Build history of the part. All positions in model axes, mm. A direction names the side the tool comes from. Coordinates: 2 decimals unless noted, no trailing zeros. Order: outer loops, then holes, each group sorted by start corner. A loop starts at its lowest first (then second) coordinate and runs counter-clockwise, first axis right, second up. Notation, with made-up numbers: M 22.5,-23 L 26.5,-23 A29 cw 26.5,8 Z; hole C 34,68 d6. An arc over 180 degrees is marked long. Write item = value, one per line. Start each with the question number.
Q1. Pull direction X, two halves, no side cores. Call faces 1 (the face through (0, 26, 1)), 2 (the face through (-19, -15, 1)), 3 (the face through (-26, 0, 1)): released by +X, released by -X, zero draft, split by the parting line, or undercut.
Q2. Band-saw the part on A-A on x = -5. Write the cut outline in (y, z), plus the area to 3 significant figures.
Q3. Band-saw the part on B-B on z = 0.65. State how many separate pieces and enclosed holes the cut face has, plus the area to 3 significant figures.
Q4. Band-saw the part on C-C on y = 8.25. Write the cut outline in (x, z).
Q5. 3-axis set-ups, long thin cutter, end or side, ignore diameter. For faces 4 (the face through (12.85, -9, 1)), 5 (the face through (0, 0, 2)): which of +Z, -Z, +X, -X, +Y, -Y reach the whole face in a straight line?
Q6. Drill centre lines: probe 1 along Y at (x, z) = (5.5, 0.2); probe 2 along Y at (x, z) = (15.25, 1.2); probe 3 along Y at (x, z) = (-13, 0.6). Where is each one in solid material? Low to high.
Q7. Band-saw the part on D-D on x = 15.25. Write the cut outline in (y, z), plus the area to 3 significant figures.
```python
from build123d import *

# Parameters (mm, degrees)
SKETCH_W     = 52
SKETCH_H     = 52
SKETCH_R     = 1.8
SKETCH_W_2   = 38
SKETCH_H_2   = 7.5
PAD_DEPTH    = 2
SKETCH001_W  = 25.7
SKETCH001_H  = 8
POCKET_DEPTH = 5


with BuildPart() as part:
    # Sketch → Pad (new body)
    with BuildSketch(Plane.XY):
        Rectangle(SKETCH_W, SKETCH_H)
        with Locations((22.25, 22.25)):
            Circle(SKETCH_R, mode=Mode.SUBTRACT)
        with Locations((22.25, -22.25)):
            Circle(SKETCH_R, mode=Mode.SUBTRACT)
        with Locations((-22.25, 22.25)):
            Circle(SKETCH_R, mode=Mode.SUBTRACT)
        with Locations((-22.25, -22.25)):
            Circle(SKETCH_R, mode=Mode.SUBTRACT)
        with Locations((15.25, 8.25)):
            Circle(SKETCH_R, mode=Mode.SUBTRACT)
        with Locations((-15.25, 8.25)):
            Circle(SKETCH_R, mode=Mode.SUBTRACT)
        with Locations((-15.25, -8.25)):
            Circle(SKETCH_R, mode=Mode.SUBTRACT)
        with Locations((15.25, -8.25)):
            Circle(SKETCH_R, mode=Mode.SUBTRACT)
        with Locations((0, 15.25)):
            Rectangle(SKETCH_W_2, SKETCH_H_2, mode=Mode.SUBTRACT)
        with Locations((0, -15.25)):
            Rectangle(SKETCH_W_2, SKETCH_H_2, mode=Mode.SUBTRACT)
    extrude(amount=PAD_DEPTH)

    # Sketch001 → Pocket (cut)
    with BuildSketch(Plane.XY.offset(2)):
        with Locations((0, -10.5)):
            Rectangle(SKETCH001_W, SKETCH001_H)
    extrude(amount=-POCKET_DEPTH, mode=Mode.SUBTRACT)


solid = part.part
```
Recorded:
q1.face_1 = zero draft
q1.face_2 = undercut
q1.face_3 = released by -X
q2.outline = M -26,0 L -19,0 L -19,2 L -26,2 Z; M -6.5,0 L 11.5,0 L 11.5,2 L -6.5,2 Z; M 19,0 L 26,0 L 26,2 L 19,2 Z
q2.area = 64.0 mm2
q3.separate_pieces = 1
q3.enclosed_holes = 10
q3.area = 1,920 mm2
q4.outline = M -26,0 L -17.05,0 L -17.05,2 L -26,2 Z; M -13.45,0 L 13.45,0 L 13.45,2 L -13.45,2 Z; M 17.05,0 L 26,0 L 26,2 L 17.05,2 Z
q5.face_4 = +Z, -Z
q5.face_5 = +Z, +X, -X, +Y, -Y
q6.probe_1 = -26 to -19, -6.5 to 11.5, 19 to 26
q6.probe_2 = -26 to -19, -11.5 to -10.05, -6.45 to 6.45, 10.05 to 11.5, 19 to 26
q6.probe_3 = -26 to -19, -11.5 to 11.5, 19 to 26
q7.outline = M -26,0 L -19,0 L -19,2 L -26,2 Z; M -11.5,0 L -10.05,0 L -10.05,2 L -11.5,2 Z; M -6.45,0 L 6.45,0 L 6.45,2 L -6.45,2 Z; M 10.05,0 L 11.5,0 L 11.5,2 L 10.05,2 Z; M 19,0 L 26,0 L 26,2 L 19,2 Z
q7.area = 59.6 mm2
